```python
from build123d import *

# Parameters (mm, degrees)
BOSS_EXTRUDE1_DEPTH = 14
BOSS_EXTRUDE2_DEPTH = 12
CUT_EXTRUDE2_DEPTH  = 6
SKETCH7_W           = 39.032004281
SKETCH7_H           = 8.14809517
CUT_EXTRUDE3_DEPTH  = 9
CUT_EXTRUDE4_DEPTH  = 14
BOSS_EXTRUDE3_DEPTH = 14


with BuildPart() as part:
    # Sketch2 → Boss-Extrude1 (new body)
    with BuildSketch(Plane(origin=(0, 0, 0), x_dir=(1, 0, 0), z_dir=(0, 1, 0))):
        Polygon((-21.65, 0), (0, 0), (0, 10), (-27.423502692, 10), (-38.810254038, -9.722431864), (-30.15, -14.722431864), align=None)
    boss_extrude1 = extrude(amount=BOSS_EXTRUDE1_DEPTH)

    # Sketch5 → Boss-Extrude2 (add)
    with BuildSketch(Plane(origin=(0, 0, 0), x_dir=(1, 0, 0), z_dir=(0, 1, 0))):
        Polygon((-38.810254038, -9.722431864), (-38.810254038, -12.031832941), (-29.417949192, -17.454482672), (-20.495299462, -2), (0, -2), (0, 0), (-21.65, 0), (-30.15, -14.722431864), align=None)
    boss_extrude2 = extrude(amount=BOSS_EXTRUDE2_DEPTH)

    # Sketch6 → Cut-Extrude2 (cut)
    with BuildSketch(Plane(origin=(0, 14, 0), x_dir=(1, 0, 0), z_dir=(0, 1, 0))):
        Polygon((-30.15, -14.722431864), (-31.708845727, -13.822431864), (-29.458845727, -9.925317547), (-33.096152423, -7.825317547), (-34.096152423, -9.557368355), (-35.82820323, -8.557368355), (-30.82820323, 0.102885683), (-29.096152423, -0.897114317), (-30.096152423, -2.629165125), (-26.458845727, -4.729165125), (-24.208845727, -0.832050808), (-22.65, -1.732050808), align=None)
    cut_extrude2 = extrude(amount=-CUT_EXTRUDE2_DEPTH, mode=Mode.SUBTRACT)

    # Sketch7 → Cut-Extrude3 (cut)
    with BuildSketch(Plane(origin=(0, 14, 0), x_dir=(1, 0, 0), z_dir=(0, 1, 0))):
        with Locations((-15.834859511, 8.074047585)):
            Rectangle(SKETCH7_W, SKETCH7_H)
    cut_extrude3 = extrude(amount=-CUT_EXTRUDE3_DEPTH, mode=Mode.SUBTRACT)

    # Mirror2: Boss-Extrude1, Boss-Extrude2, Cut-Extrude2, Cut-Extrude3 across plane
    add(boss_extrude1.mirror(Plane(origin=(0, 0, 0), x_dir=(0, 0, 1), z_dir=(1, 0, 0))))
    add(boss_extrude2.mirror(Plane(origin=(0, 0, 0), x_dir=(0, 0, 1), z_dir=(1, 0, 0))))
    add(cut_extrude2.mirror(Plane(origin=(0, 0, 0), x_dir=(0, 0, 1), z_dir=(1, 0, 0))), mode=Mode.SUBTRACT)
    add(cut_extrude3.mirror(Plane(origin=(0, 0, 0), x_dir=(0, 0, 1), z_dir=(1, 0, 0))), mode=Mode.SUBTRACT)

    # Sketch8 → Cut-Extrude4 (cut)
    with BuildSketch(Plane(origin=(0, 14, 0), x_dir=(1, 0, 0), z_dir=(0, 1, 0))):
        Polygon((-10, -2), (-4.226497308, 8), (4.226497308, 8), (10, -2), align=None)
    extrude(amount=-CUT_EXTRUDE4_DEPTH, mode=Mode.SUBTRACT)

    # Sketch9 → Boss-Extrude3 (add)
    with BuildSketch(Plane(origin=(0, 14, 0), x_dir=(1, 0, 0), z_dir=(0, 1, 0))):
        Polygon((-13.464101615, 4), (-7.690598923, 14), (7.690598923, 14), (13.464101615, 4), (6.535898385, 4), (4.226497308, 8), (-4.226497308, 8), (-6.535898385, 4), align=None)
    extrude(amount=-BOSS_EXTRUDE3_DEPTH)


solid = part.part
```
For this review, take the finished solid that the model builds, in its own axes (mm). A direction names the side the tool comes from. Give positions to 0.01 mm unless a question says otherwise; leave off trailing zeros. Order: outer loops, then holes, each group sorted by start corner. A loop starts at its lowest first (then second) coordinate and runs counter-clockwise, first axis right, second up.
1) Wall thickness on line 1 (X direction, y = 10, z = 5.5); line 2 (X direction, y = 8.5, z = 6); line 3 (Z direction, x = 32, y = 9.5): over which ranges is each line inside the solid? List them lowest first.
2) Take a section at C-C (y = 1.5). Give the boundary of the cut face in (x, z).
3) For faces 4 (the face through (-24, 12, 7)), 5 (the face through (-29.974, 11.042, 0.39)), 6 (the face through (15, 6, 2)), list the 3-axis set-ups (+Z, -Z, +X, -X, +Y, -Y) from which the entire face can be reached by the end or side of a thin tool; tool diameter is ignored.
4) Insertion check: pin 1 (5 mm diameter, centred on x = 23.5, z = 12, fed in from +Y); pin 2 (3 mm diameter, centred on x = -17, y = 7.5, fed in from +Z); pin 3 (5 mm diameter, centred on x = 14.5, y = 12, fed in from -Z); pin 4 (8.5 mm diameter, centred on x = -29.5, z = 11, fed in from +Y). Each pin has a flat end and moves straight along its axis. Give the tip position at first contact, or say it passes through.
5) The part is to be moulded in two halves that separate along X. For faces 1 (the face through (-19, 2, -10)), 2 (the face through (-38.81, 6, 11)), 3 (the face through (-30.6, 11, 11.9)), say which applies: released by +X, released by -X, zero draft, split by the parting line, or undercut.
6) Take a section at B-B (x = -19). Give the boundary of the cut face in (y, z).
7) Take a section at D-D (z = -6). Give the boundary of the cut face in (x, y).
8) Take a section at A-A (z = -1). Give the boundary of the cut face in (x, y).
Derived:
1. line 1: x = -36.37 to -34.06, -24.83 to -22.52, 22.52 to 24.83, 34.06 to 36.37
1. line 2: x = -36.66 to -34.35, -25.11 to -22.8, 22.8 to 25.11, 34.35 to 36.66
1. line 3: z = -2.07 to 1.93, 8.46 to 15.96
2. outline: (-38.81, 9.72) - (-27.42, -10) - (-10, -10) - (-7.69, -14) - (7.69, -14) - (10, -10) - (27.42, -10) - (38.81, 9.72) - (38.81, 12.03) - (29.42, 17.45) - (20.5, 2) - (10, 2) - (4.23, -8) - (-4.23, -8) - (-10, 2) - (-20.5, 2) - (-29.42, 17.45) - (-38.81, 12.03) - close
3. face 4: +Z, +Y
3. face 5: +Y
3. face 6: +Z, +Y, -Y
4. pin 1: stops at y = 12
4. pin 2: stops at z = 2
4. pin 3: stops at z = -6.54
4. pin 4: stops at y = 14
5. face 1: zero draft
5. face 2: released by -X
5. face 3: undercut
6. outline: (0, -10) - (5, -10) - (5, -4) - (14, -4) - (14, 0) - (12, 0) - (12, 2) - (0, 2) - close
7. outline: (-29.73, 0) - (-5.38, 0) - (-5.38, 14) - (-12.31, 14) - (-12.31, 5) - (-29.73, 5) - close; (5.38, 0) - (29.73, 0) - (29.73, 5) - (12.31, 5) - (12.31, 14) - (5.38, 14) - close
8. outline: (-32.62, 0) - (-8.27, 0) - (-8.27, 14) - (-32.62, 14) - close; (8.27, 0) - (32.62, 0) - (32.62, 14) - (8.27, 14) - close
